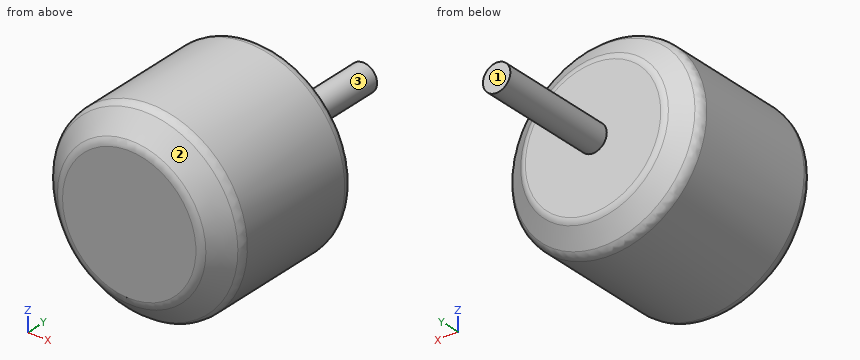
Autodesk Inventor part; units mm, degrees
ref_plane "YZ Plane" through (0, 0, 0) normal (1, 0, 0) x (0, 1, 0)
ref_plane "XZ Plane" through (0, 0, 0) normal (0, 1, 0) x (-1, 0, 0)
ref_plane "XY Plane" through (0, 0, 0) normal (0, 0, 1) x (1, 0, 0)
sketch "Sketch1" plane through (0, 0, 0) normal (0, 0, 1) x (1, 0, 0)
  line L0 (0, 43.18) -> (0, 0)
  line L1 (-10.3763, 25.4) -> (-2, 25.4)
  line L2 (-2, 25.4) -> (-2, 43.18)
  line L3 (-2, 43.18) -> (0, 43.18)
  line L4 (0, 0) -> (-10.3763, 0)
  line L5 (-10.3763, 0) -> (-13.97, 3.466)
  line L6 (-13.97, 3.466) -> (-13.97, 22.9252)
  line L7 (-13.97, 22.9252) -> (-10.3763, 25.4)
  point P0 (0, 21.59)
  dimension "d18" = 2
  dimension "d19" = 17.78
  dimension "d23" = 25.4
  dimension "d25" = 13.97
revolve "Revolution1" add sketch "Sketch1" angle 360 about axis through (0, 43.18, 0) along (0, -1, 0)
fillet "Fillet3" radius 1.5875 1 edges at (10.3763, 25.4, 0)
fillet "Fillet4" radius 1.5875 1 edges at (13.97, 22.9252, 0)
fillet "Fillet5" radius 1.5875 2 edges at (13.97, 3.466, 0) (10.3763, 0, 0)
properties part number "MotorTop"
Input: part model. Units: mm. Frame: model coordinates. Face numbers are marked on the shaded views. Round coordinates to 2 decimals unless told otherwise and drop trailing zeros. Loops run counter-clockwise (first coordinate to the right, second up) from the corner with the lowest first, then second, coordinate; pieces in that order, holes last. Notation, with made-up numbers: (51, -1.5) -> (95, -1.5) arc R20 cw to (95, 3.5) -> close; hole circle Ø6 at (49.25, 86.25). An arc over 180 degrees is marked (long way). Answer as a JSON object with one key per item and string values. Group by question number.
1) Section query A-A on y = 31.5. Output: boundary loops of the cut face in (x, z).
2) Ray query, L1, parallel to X at y = 29, z = 0; L2, parallel to Y at x = 4.25, z = 2.25; L3, parallel to Y at x = -1.5, z = -10.5. Return the intervals inside material, ascending.
3) Section query B-B on y = 7. Output: boundary loops of the cut face in (x, z).
4) Draft query along Y for the marked faces 1, 2 and 3. Return one class per face: +Y half, -Y half, draft (parallel to the pull), parting line (faces both ways), or undercut.
5) Pin query (flat end, axial travel): pin 1 (4 mm diameter, centred on x = -7.5, y = 27, fed in from +Z); pin 2 (3 mm diameter, centred on x = -6.5, y = 8.5, fed in from +Z); pin 3 (2 mm diameter, centred on x = -7.5, y = 8, fed in from +Z). Return the tip coordinate at first contact, or that it passes through.
Reply:
{
 "1": {"outline": "circle Ø4 at (0, 0)"},
 "2": {"L1": "x = -2 to 2", "L2": "y = 0 to 25.4", "L3": "y = 0.26 to 25.23"},
 "3": {"outline": "circle Ø27.94 at (0, 0)"},
 "4": {"face 1": "+Y half", "face 2": "-Y half", "face 3": "draft"},
 "5": {"pin 1": "stops at z = 8.36", "pin 2": "stops at z = 13.04", "pin 3": "stops at z = 12.37"}
}
